For this review, take the finished solid that the model builds, in its own axes (mm). Face numbers are marked on the shaded views. A direction names the side the tool comes from. Coordinates: 2 decimals unless noted, no trailing zeros. Loops run counter-clockwise (first coordinate to the right, second up) from the corner with the lowest first, then second, coordinate; pieces in that order, holes last. Notation, with made-up numbers: (-37.75, 49) - (-12.75, 49) arc R15 cw to (-12.75, 73) - close; hole circle Ø10 at (85.5, 0). An arc over 180 degrees is marked (long way). One line per item, written item: value. Start each with the question number.
1. Take a section at A-A, the plane x = 8. State the section outline as (y, z) points, and give its area (3 significant figures).
2. Take a section at D-D, the plane y = -46. State the section outline as (x, z) points, and give its area (3 significant figures).
3. Take a section at C-C, the plane z = -126. State the section outline as (x, y) points, and give its area (3 significant figures).
4. The part is to be moulded in two halves that separate along Y. For the marked faces 1, 2, 3 and 4, say which applies: released by +Y, released by -Y, zero draft, split by the parting line, or undercut.
5. For the marked faces 5, 6, 7 and 8, list the 3-axis set-ups (+Z, -Z, +X, -X, +Y, -Y) from which the entire face can be reached by the end or side of a thin tool; tool diameter is ignored.
6. Insertion check: pin 1 (1.5 mm diameter, centred on x = -21.5, z = -95, fed in from +Y); pin 2 (12 mm diameter, centred on x = 12, z = -83.5, fed in from +Y); pin 3 (1.5 mm diameter, centred on x = 19, z = -95, fed in from -Y). Each pin has a flat end and moves straight along its axis. Give the tip position at first contact, or say it passes through.
7. Take a section at B-B, the plane y = -5. State the section outline as (x, z) points, and give its area (3 significant figures).
8. To check wall thickness, follow line 1 (X direction, y = -5, z = -117); line 2 (X direction, y = -40, z = -63.75); line 3 (Y direction, x = 39, z = -66). State the ranges of each line that lie inside material, in increasing order. Write a range as from..to.
```python
from build123d import *

# Parameters (mm, degrees)
CYLINDER001_R          = 3
CYLINDER001_DEPTH      = 20
CYLINDER_R             = 10
CYLINDER_DEPTH         = 50
PAD008_DEPTH           = 92
CUT002_PLACEMENT_ANGLE = 90


with BuildPart() as cylinder001:
    # Cylinder001 → Cylinder001 (new body)
    with BuildSketch(Plane(origin=(-31, -46, 34), x_dir=(1, 0, 0), z_dir=(0, 0, 1))):
        Circle(CYLINDER001_R)
    extrude(amount=CYLINDER001_DEPTH)


with BuildPart() as cylinder:
    # Cylinder → Cylinder (new body)
    with BuildSketch(Plane(origin=(4, -44, -38), x_dir=(1, 0, 0), z_dir=(0, 0, 1))):
        Circle(CYLINDER_R)
    extrude(amount=CYLINDER_DEPTH)


with BuildPart() as stand001:
    # Sketch009 → Pad008 (new body)
    with BuildSketch(Plane.XZ):
        Polygon((45, -27.665999), (-45, -27.665999), (-45, -5.665999), (-5, 36.334001), (-75, 36.334001), (-75, 52.334001), (15, 52.334001), (15, 36.334001), (-25, -5.665999), (45, -5.665999), align=None)
    extrude(amount=PAD008_DEPTH)

    # Cut001: cut Cylinder
    add(cylinder.part, mode=Mode.SUBTRACT)

    # Cut002: cut Cylinder001
    add(cylinder001.part, mode=Mode.SUBTRACT)


with BuildPart() as stand001_1:
    # Cut002 placement: moved
    add(stand001.part.moved(Location((-44, -9, -104))).rotate(Axis((-44, -9, -104), (0, 0, 1)), CUT002_PLACEMENT_ANGLE))


solid = stand001_1.part
```
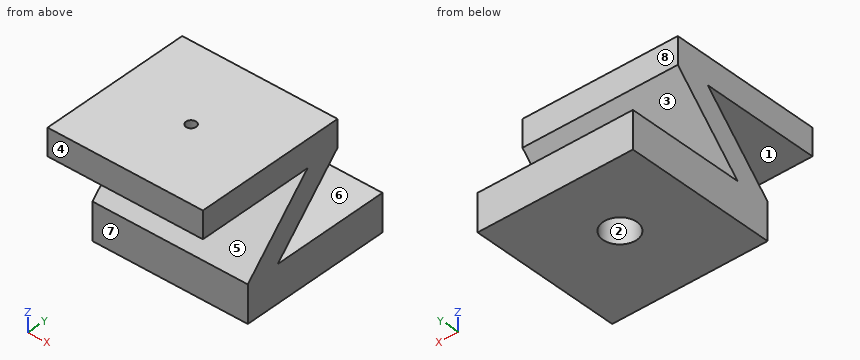
Solutions:
1. outline: (-84, -67.67) - (-14, -67.67) - (-54, -109.67) - (-54, -131.67) - (-11, -131.67) - (-11, -109.67) - (-34, -109.67) - (6, -67.67) - (6, -51.67) - (-84, -51.67) - close; (1, -131.67) - (36, -131.67) - (36, -109.67) - (1, -109.67) - close
1. area: 4,000 mm2
2. outline: (-44, -131.67) - (48, -131.67) - (48, -101.27) - (-44, -101.27) - close; (-44, -67.67) - (48, -67.67) - (48, -51.67) - (-44, -51.67) - close
2. area: 4,270 mm2
3. outline: (-44, -54) - (48, -54) - (48, 36) - (-44, 36) - close; hole circle Ø20 at (0, -5)
3. area: 7,970 mm2
4. face 1: zero draft
4. face 2: undercut
4. face 3: released by +Y
4. face 4: released by -Y
5. face 5: +X, -X, -Y
5. face 6: +X, -X, +Y
5. face 7: -Z, +X, -X, -Y
5. face 8: +Z, +X, -X, +Y
6. pin 1: y = -19.32
6. pin 2: y = -3.37
6. pin 3: y = -40.75
7. outline: (-44, -131.67) - (-10, -131.67) - (-10, -109.67) - (-44, -109.67) - close; (-44, -79.22) - (48, -79.22) - (48, -51.67) - (-44, -51.67) - close; (10, -131.67) - (48, -131.67) - (48, -109.67) - (10, -109.67) - close
7. area: 4,120 mm2
8. line 1: -44..-10, 10..48
8. line 2: -44..-1, 5..48
8. line 3: -84..6
